Autodesk Inventor part; units mm, degrees
ref_plane "C1_XY" through (0, 0, 0) normal (0, 0, 1) x (1, 0, 0)
ref_plane "C1_YZ" through (0, 0, 0) normal (1, 0, 0) x (0, 1, 0)
ref_plane "C1_ZX" through (0, 0, 0) normal (0, 1, 0) x (0, 0, 1)
sketch "Sketch_60" plane through (0, 0, 0) normal (0, 0, 1) x (1, 0, 0)
  arc A0 (-30, -27) -> (-27, -30) centre (-27, -27) ccw
  line L0 (-27, -30) -> (-5, -30)
  line L1 (-5, -30) -> (-5, -24)
  line L2 (-5, -24) -> (-10, -24)
  line L3 (-10, -24) -> (-10, -19.6167)
  line L4 (-10, -19.6167) -> (-7.3833, -17)
  line L5 (-7.3833, -17) -> (-3.3464, -17)
  line L6 (-3.3464, -17) -> (-3, -16.8)
  line L7 (-3, -16.8) -> (-2.6536, -17)
  line L8 (-2.6536, -17) -> (-1.2124, -17)
  line L9 (-1.2124, -17) -> (0, -16.3)
  line L10 (0, -16.3) -> (1.2124, -17)
  line L11 (1.2124, -17) -> (2.6536, -17)
  line L12 (2.6536, -17) -> (3, -16.8)
  line L13 (3, -16.8) -> (3.3464, -17)
  line L14 (3.3464, -17) -> (7.3833, -17)
  line L15 (7.3833, -17) -> (10, -19.6167)
  line L16 (10, -19.6167) -> (10, -24)
  line L17 (10, -24) -> (5, -24)
  line L18 (5, -24) -> (5, -30)
  line L19 (5, -30) -> (27, -30)
  arc A1 (27, -30) -> (30, -27) centre (27, -27) ccw
  line L20 (30, -27) -> (30, -5)
  line L21 (30, -5) -> (24, -5)
  line L22 (24, -5) -> (24, -10)
  line L23 (24, -10) -> (19.6167, -10)
  line L24 (19.6167, -10) -> (17, -7.3833)
  line L25 (17, -7.3833) -> (17, -3.3464)
  line L26 (17, -3.3464) -> (16.8, -3)
  line L27 (16.8, -3) -> (17, -2.6536)
  line L28 (17, -2.6536) -> (17, -1.2124)
  line L29 (17, -1.2124) -> (16.3, 0)
  line L30 (16.3, 0) -> (17, 1.2124)
  line L31 (17, 1.2124) -> (17, 2.6536)
  line L32 (17, 2.6536) -> (16.8, 3)
  line L33 (16.8, 3) -> (17, 3.3464)
  line L34 (17, 3.3464) -> (17, 7.3833)
  line L35 (17, 7.3833) -> (19.6167, 10)
  line L36 (19.6167, 10) -> (24, 10)
  line L37 (24, 10) -> (24, 5)
  line L38 (24, 5) -> (30, 5)
  line L39 (30, 5) -> (30, 27)
  arc A2 (30, 27) -> (27, 30) centre (27, 27) ccw
  line L40 (27, 30) -> (5, 30)
  line L41 (5, 30) -> (5, 24)
  line L42 (5, 24) -> (10, 24)
  line L43 (10, 24) -> (10, 19.6167)
  line L44 (10, 19.6167) -> (7.3833, 17)
  line L45 (7.3833, 17) -> (3.3464, 17)
  line L46 (3.3464, 17) -> (3, 16.8)
  line L47 (3, 16.8) -> (2.6536, 17)
  line L48 (2.6536, 17) -> (1.2124, 17)
  line L49 (1.2124, 17) -> (0, 16.3)
  line L50 (0, 16.3) -> (-1.2124, 17)
  line L51 (-1.2124, 17) -> (-2.6536, 17)
  line L52 (-2.6536, 17) -> (-3, 16.8)
  line L53 (-3, 16.8) -> (-3.3464, 17)
  line L54 (-3.3464, 17) -> (-7.3833, 17)
  line L55 (-7.3833, 17) -> (-10, 19.6167)
  line L56 (-10, 19.6167) -> (-10, 24)
  line L57 (-10, 24) -> (-5, 24)
  line L58 (-5, 24) -> (-5, 30)
  line L59 (-5, 30) -> (-27, 30)
  arc A3 (-27, 30) -> (-30, 27) centre (-27, 27) ccw
  line L60 (-30, 27) -> (-30, 5)
  line L61 (-30, 5) -> (-24, 5)
  line L62 (-24, 5) -> (-24, 10)
  line L63 (-24, 10) -> (-19.6167, 10)
  line L64 (-19.6167, 10) -> (-17, 7.3833)
  line L65 (-17, 7.3833) -> (-17, 3.3464)
  line L66 (-17, 3.3464) -> (-16.8, 3)
  line L67 (-16.8, 3) -> (-17, 2.6536)
  line L68 (-17, 2.6536) -> (-17, 1.2124)
  line L69 (-17, 1.2124) -> (-16.3, 0)
  line L70 (-16.3, 0) -> (-17, -1.2124)
  line L71 (-17, -1.2124) -> (-17, -2.6536)
  line L72 (-17, -2.6536) -> (-16.8, -3)
  line L73 (-16.8, -3) -> (-17, -3.3464)
  line L74 (-17, -3.3464) -> (-17, -7.3833)
  line L75 (-17, -7.3833) -> (-19.6167, -10)
  line L76 (-19.6167, -10) -> (-24, -10)
  line L77 (-24, -10) -> (-24, -5)
  line L78 (-24, -5) -> (-30, -5)
  line L79 (-30, -5) -> (-30, -27)
  circle A4 centre (20, 20) radius 3.5
  circle A5 centre (20, -20) radius 3.5
  circle A6 centre (-20, 20) radius 3.5
  circle A7 centre (-20, -20) radius 3.5
extrude "Extrusion1" add sketch "Sketch_60" against normal blind 2667
sketch "Sketch2" plane through (0, 0, -2667) normal (0, 0, -1) x (-1, 0, 0)
  point P0 (0, 0)
hole "Hole1" at (0, 0, -2667) direction (0, 0, 1) diameter 10.5 depth 1000
ref_plane "C1_XY" through (0, 0, 0) normal (0, 0, 1) x (1, 0, 0)
ref_plane "C1_YZ" through (0, 0, 0) normal (1, 0, 0) x (0, 1, 0)
ref_plane "C1_ZX" through (0, 0, 0) normal (0, 1, 0) x (0, 0, 1)
ref_plane "to_frame_cap1_XY" through (0, 0, 0) normal (0, 0, 1) x (1, 0, 0)
ref_plane "to_frame_cap1_YZ" through (0, 0, 0) normal (1, 0, 0) x (0, 1, 0)
ref_plane "to_frame_cap1_ZX" through (0, 0, 0) normal (0, 1, 0) x (0, 0, 1)
ref_plane "to_frame_cap2_XY" through (0, 0, -1000) normal (0, 0, -1) x (1, 0, 0)
ref_plane "to_frame_cap2_YZ" through (0, 0, -1000) normal (1, 0, 0) x (0, -1, 0)
ref_plane "to_frame_cap2_ZX" through (0, 0, -1000) normal (0, -1, 0) x (0, 0, -1)
properties part number "GFS8-6060-1000"
Geometry check sheet. Reference: the model listing, model coordinates, mm. Coordinates: 2 decimals unless noted, no trailing zeros. Answer in a Markdown table with one row per item. Add a question column.
1. Material ranges on L1, parallel to Y at x = 21.5, z = -1672; L2, parallel to X at y = -7, z = -1149; L3, parallel to Y at x = -20, z = -2044, recorded low to high. Write a range as [from, to].
2. Gauge pin test, flat ends, axial feed: pin 1 Ø0.7 at (x, z) = (-2, -1347.5) entering from -Y; pin 2 Ø0.7 at (y, z) = (2, -1834) entering from +X; pin 3 Ø6.5 at (x, y) = (-20, 20) entering from +Z (1 decimal); pin 4 Ø5 at (x, y) = (-1.5, -2) entering from -Z. Record the tip position at first contact, or that the pin passes through.
3. Section check A-A (z = -2357). Give the number of separate pieces and of enclosed holes in the cut face, plus the area to 3 significant figures.
Data:
| question | item | result |
|---|---|---|
| 1 | L1 | y = [-30, -23.16], [-16.84, -10], [10, 16.84], [23.16, 30] |
| 1 | L2 | x = [-30, -24], [-17, 17], [24, 30] |
| 1 | L3 | y = [-30, -23.5], [-16.5, -10], [10, 16.5], [23.5, 30] |
| 2 | pin 1 | stops at y = -17 |
| 2 | pin 2 | stops at x = 17 |
| 2 | pin 3 | passes through |
| 2 | pin 4 | stops at z = -1667 |
| 3 | separate pieces | 1 |
| 3 | enclosed holes | 5 |
| 3 | area | 2,580 mm² |
